Drawing for the job (mm, zero at the part's lowest x, y, z). Round coordinates to 2 decimals unless told otherwise and drop trailing zeros. Write each loop counter-clockwise with the first axis right and the second up, starting at its lowest first coordinate (ties: lowest second). Pieces come first, ordered by that corner, then holes.
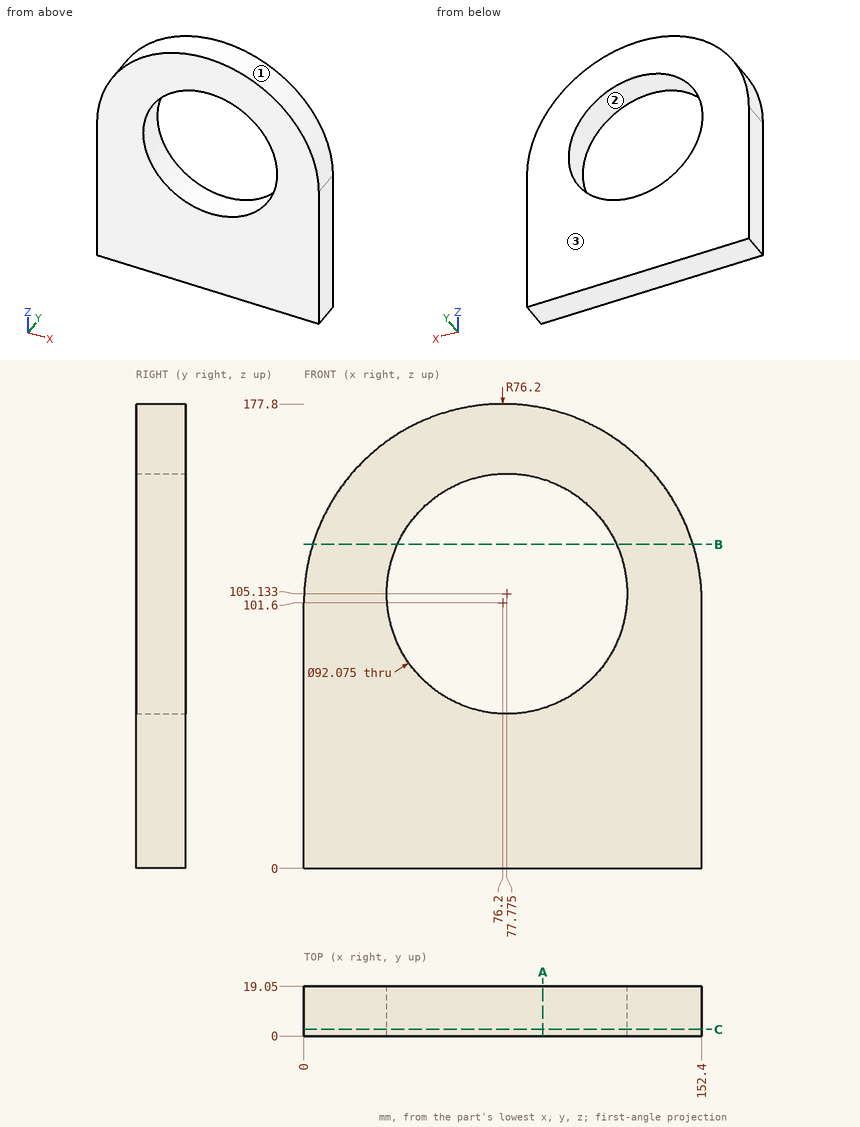
Q1. Drop flat-ended pins along their axis: P1, Ø2, axis at x = 59, y = 15.5, coming from the +Z side; P2, Ø4, axis at x = 32.5, y = 10, coming from the +Z side; P3, Ø1, axis at x = 76.5, y = 17, coming from the +Z side. Give the stop position or say it passes through.
Q2. Saw through at C-C, the plane y = 2.5. Write the cut outline in (x, z) (1 decimal).
Q3. Saw through at B-B, the plane z = 124. Write the cut outline in (x, y), and give its area (4 significant figures).
Q4. Wall check: line 1 (X direction, y = 4.5, z = 118.5); line 2 (Z direction, x = 118, y = 2) (1 decimal); line 3 (Z direction, x = 78, y = 3.25). Give the ranges that are in metal, low to high.
Q5. Saw through at A-A, the plane x = 91.5. Write the cut outline in (y, z).
Q6. Two-plate mould, pull along X, no slides. Class the marked faces 1, 2 and 3: released by +X, released by -X, zero draft, split by the parting line, or undercut.
Computed:
1. P1: stops at z = 176.06
1. P2: stops at z = 165.38
1. P3: stops at z = 177.8
2. outline: (0, 0) - (152.4, 0) - (152.4, 101.6) arc R76.2 ccw to (0, 101.6) - close; hole circle Ø92.1 at (77.8, 105.1)
3. outline: (3.37, 0) - (35.78, 0) - (35.78, 19.05) - (3.37, 19.05) - close; (119.77, 0) - (149.03, 0) - (149.03, 19.05) - (119.77, 19.05) - close
3. area: 1,175 mm2
4. line 1: x = 1.9 to 33.72, 121.83 to 150.5
4. line 2: z = 0 to 82.7, 127.5 to 165.3
4. line 3: z = 0 to 59.1, 151.17 to 177.78
5. outline: (0, 0) - (19.05, 0) - (19.05, 61.19) - (0, 61.19) - close; (0, 149.08) - (19.05, 149.08) - (19.05, 176.25) - (0, 176.25) - close
6. face 1: split by the parting line
6. face 2: undercut
6. face 3: zero draft
